Read the model definition and answer for the solid it produces. Units are mm, in the model's axes. A direction names the side the tool comes from. Round coordinates to 2 decimals unless told otherwise and drop trailing zeros. Order: outer loops, then holes, each group sorted by start corner. A loop starts at its lowest first (then second) coordinate and runs counter-clockwise, first axis right, second up. Notation, with made-up numbers: (68.25, 66.5) -> (92.25, 66.5) arc R15 ccw to (92.25, 76.5) -> close; hole circle Ø5 at (-1, 7.5). An arc over 180 degrees is marked (long way). Answer as a JSON object with one key per item and string values. Group by question number.
Item 1: Section B-B, the plane z = 15 is taken. Write down the section's boundary in (x, y), plus the area to 3 significant figures.
Item 2: Section D-D, the plane x = -20 is taken. Write down the section's boundary in (y, z), plus the area to 3 significant figures.
Item 3: Section C-C, the plane y = -17.5 is taken. Write down the section's boundary in (x, z), plus the area to 3 significant figures.
Item 4: Section A-A, the plane y = 0 is taken. Write down the section's boundary in (x, z).
Item 5: For faces 1 (the flat face through (22.86, 0, 1)), 2 (the flat face through (10.499, -4, 16)), 3 (the flat face through (-17, 1.907, 13)), determine the directions among +Z, -Z, +X, -X, +Y, -Y from which every point of the face is accessible in a straight line to the end or side of a thin tool.
Item 6: The mould has two halves that part along Y. Classify faces 4 (the flat face through (-10.01, 3.03, 6.26)), 5 (the flat face through (-2, -11, 19.05)), 6 (the flat face through (-22.399, -11, 13)): pulls with the +Y half, pulls with the -Y half, needs draft (parallel to the pull), parting line crosses it, or undercut.
Item 7: Consider probe 1 along X at (y, z) = (-11.5, 18); probe 2 along X at (y, z) = (0, 9); probe 3 along X at (y, z) = (-9.25, 18). Determine where each line is inside the solid, lowest interval first. Write a range as from..to.
Item 8: Given P1, Ø1, axis at x = -0.5, z = 0.5, coming from the +Y side; P2, Ø1.5, axis at x = 18.5, y = 1, coming from the -Z side; P3, Ø1.9, axis at x = 4, z = 15, coming from the +Y side, each flat-ended and moving along its own axis, determine where each tip first touches the part or whether it passes through.
from build123d import *

# Parameters (mm, degrees)
BOSS_EXTRUDE1_DEPTH = 12.7
SKETCH2_W           = 12.7
SKETCH2_H           = 12.7
BOSS_EXTRUDE2_DEPTH = 22.22735
BOSS_EXTRUDE3_DEPTH = 12.7
SKETCH4_W           = 12.7
SKETCH4_H           = 12.7
BOSS_EXTRUDE4_DEPTH = 22.22735
BOSS_EXTRUDE5_DEPTH = 12.7
BOSS_EXTRUDE6_DEPTH = 6.35
CUT_EXTRUDE1_DEPTH  = 12.7
SKETCH9_W           = 10.16
SKETCH9_H           = 5.08
SKETCH9_W_2         = 5.08
SKETCH9_H_2         = 10.16
CUT_EXTRUDE2_DEPTH  = 2


with BuildPart() as part:
    # Sketch1 → Boss-Extrude1 (new body)
    with BuildSketch(Plane.XY):
        with BuildLine():
            Line((10.499121608, 3.177349953), (9.526676859, 2.883058926))
            ThreePointArc((9.526676859, 2.883058926), (0, -9.953371325), (-9.526676859, 2.883058926))
            Line((-9.526676859, 2.883058926), (-10.499121608, 3.177349953))
            ThreePointArc((-10.499121608, 3.177349953), (-10.851172075, 1.605980037), (-10.969371325, 0))
            Line((-10.969371325, 0), (-10.969371325, -19.05))
            Line((-10.969371325, -19.05), (-23.669371325, -19.05))
            Line((-23.669371325, -19.05), (-23.669371325, -25.4))
            Line((-23.669371325, -25.4), (23.669371325, -25.4))
            Line((23.669371325, -25.4), (23.669371325, -19.05))
            Line((23.669371325, -19.05), (10.969371325, -19.05))
            Line((10.969371325, -19.05), (10.969371325, 0))
            ThreePointArc((10.969371325, 0), (10.851172075, 1.605980037), (10.499121608, 3.177349953))
        make_face()
    extrude(amount=BOSS_EXTRUDE1_DEPTH)

    # Sketch2 → Boss-Extrude2 (add)
    with BuildSketch(Plane(origin=(0, -19.05, 0), x_dir=(1, 0, 0), z_dir=(0, 1, 0))):
        with Locations((17.319371325, -6.35)):
            Rectangle(SKETCH2_W, SKETCH2_H)
    extrude(amount=BOSS_EXTRUDE2_DEPTH)

    # Sketch3 → Boss-Extrude3 (add, through all)
    with BuildSketch(Plane(origin=(0, 0, 0), x_dir=(-1, 0, 0), z_dir=(0, 0, -1))):
        with BuildLine():
            Line((-10.969371325, 0), (-10.969371325, 3.177349953))
            Line((-10.969371325, 3.177349953), (-10.499121608, 3.177349953))
            ThreePointArc((-10.499121608, 3.177349953), (-10.851172075, 1.605980037), (-10.969371325, 0))
        make_face()
    extrude(amount=-BOSS_EXTRUDE3_DEPTH)

    # Sketch4 → Boss-Extrude4 (add)
    with BuildSketch(Plane(origin=(0, -19.05, 0), x_dir=(1, 0, 0), z_dir=(0, 1, 0))):
        with Locations((-17.319371325, -6.35)):
            Rectangle(SKETCH4_W, SKETCH4_H)
    extrude(amount=BOSS_EXTRUDE4_DEPTH)

    # Sketch5 → Boss-Extrude5 (add, through all)
    with BuildSketch(Plane(origin=(0, 0, 0), x_dir=(-1, 0, 0), z_dir=(0, 0, -1))):
        with BuildLine():
            Line((10.969371325, 3.177349953), (10.969371325, 0))
            ThreePointArc((10.969371325, 0), (10.851172075, 1.605980037), (10.499121608, 3.177349953))
            Line((10.499121608, 3.177349953), (10.969371325, 3.177349953))
        make_face()
    extrude(amount=-BOSS_EXTRUDE5_DEPTH)

    # Sketch6 → Boss-Extrude6 (add)
    with BuildSketch(Plane.XY.offset(12.7)):
        Polygon((-23.669371325, 3.177349953), (-23.669371325, -25.4), (23.669371325, -25.4), (23.669371325, 3.177349953), (10.499121608, 3.177349953), (10.499121608, -10.792650047), (-10.499121608, -10.792650047), (-10.499121608, 3.177349953), align=None)
    extrude(amount=BOSS_EXTRUDE6_DEPTH)

    # Sketch7 → Cut-Extrude1 (cut)
    with BuildSketch(Plane.XY.offset(19.05)):
        Polygon((-11.769121608, 1.907349953), (-22.399371325, 1.907349953), (-22.399371325, -24.13), (22.399371325, -24.13), (22.399371325, 1.907349953), (11.769121608, 1.907349953), (11.769121608, -12.062650047), (-11.769121608, -12.062650047), align=None)
    extrude(amount=-CUT_EXTRUDE1_DEPTH, mode=Mode.SUBTRACT)

    # Sketch9 → Cut-Extrude2 (cut)
    with BuildSketch(Plane(origin=(0, 0, 0), x_dir=(-1, 0, 0), z_dir=(0, 0, -1))):
        with Locations((-17.78, 0)):
            Rectangle(SKETCH9_W, SKETCH9_H)
        with Locations((0, -17.78)):
            Rectangle(SKETCH9_W_2, SKETCH9_H_2)
    extrude(amount=-CUT_EXTRUDE2_DEPTH, mode=Mode.SUBTRACT)


solid = part.part
Values found:
{
 "1": {"outline": "(-23.67, -25.4) -> (23.67, -25.4) -> (23.67, 3.18) -> (10.5, 3.18) -> (10.5, -10.79) -> (-10.5, -10.79) -> (-10.5, 3.18) -> (-23.67, 3.18) -> close; hole (-22.4, -24.13) -> (22.4, -24.13) -> (22.4, 1.91) -> (11.77, 1.91) -> (11.77, -12.06) -> (-11.77, -12.06) -> (-11.77, 1.91) -> (-22.4, 1.91) -> close", "area": "222 mm2"},
 "2": {"outline": "(-25.4, 0) -> (3.18, 0) -> (3.18, 19.05) -> (1.91, 19.05) -> (1.91, 6.35) -> (-24.13, 6.35) -> (-24.13, 19.05) -> (-25.4, 19.05) -> close", "area": "214 mm2"},
 "3": {"outline": "(-23.67, 0) -> (-2.54, 0) -> (-2.54, 2) -> (2.54, 2) -> (2.54, 0) -> (23.67, 0) -> (23.67, 19.05) -> (22.4, 19.05) -> (22.4, 6.35) -> (-22.4, 6.35) -> (-22.4, 19.05) -> (-23.67, 19.05) -> close", "area": "323 mm2"},
 "4": {"outline": "(-23.67, 0) -> (-9.95, 0) -> (-9.95, 12.7) -> (-10.5, 12.7) -> (-10.5, 19.05) -> (-11.77, 19.05) -> (-11.77, 6.35) -> (-22.4, 6.35) -> (-22.4, 19.05) -> (-23.67, 19.05) -> close; (9.95, 0) -> (12.7, 0) -> (12.7, 2) -> (22.86, 2) -> (22.86, 0) -> (23.67, 0) -> (23.67, 19.05) -> (22.4, 19.05) -> (22.4, 6.35) -> (11.77, 6.35) -> (11.77, 19.05) -> (10.5, 19.05) -> (10.5, 12.7) -> (9.95, 12.7) -> close"},
 "5": {"face 1": "-Z", "face 2": "+Z, +Y", "face 3": "+Z"},
 "6": {"face 4": "pulls with the +Y half", "face 5": "needs draft", "face 6": "undercut"},
 "7": {"probe 1": "-23.67..-22.4, -11.77..11.77, 22.4..23.67", "probe 2": "-23.67..-22.4, -11.77..-9.95, 9.95..11.77, 22.4..23.67", "probe 3": "-23.67..-22.4, -11.77..-10.5, 10.5..11.77, 22.4..23.67"},
 "8": {"P1": "y = -9.9", "P2": "z = 2", "P3": "y = -10.79"}
}
